Answer from the drawing. Dimensions are ordinates in mm from the lowest x, y and z of the part. Coordinates: 2 decimals unless noted, no trailing zeros. Write each loop counter-clockwise with the first axis right and the second up, starting at its lowest first coordinate (ties: lowest second). Pieces come first, ordered by that corner, then holes. Notation, with made-up numbers: (74, 28) - (131, 28) arc R17 cw to (131, 57) - close; hole circle Ø9 at (79.5, 4). An arc over 180 degrees is marked (long way). Return JSON: item names as keys, results as strings.
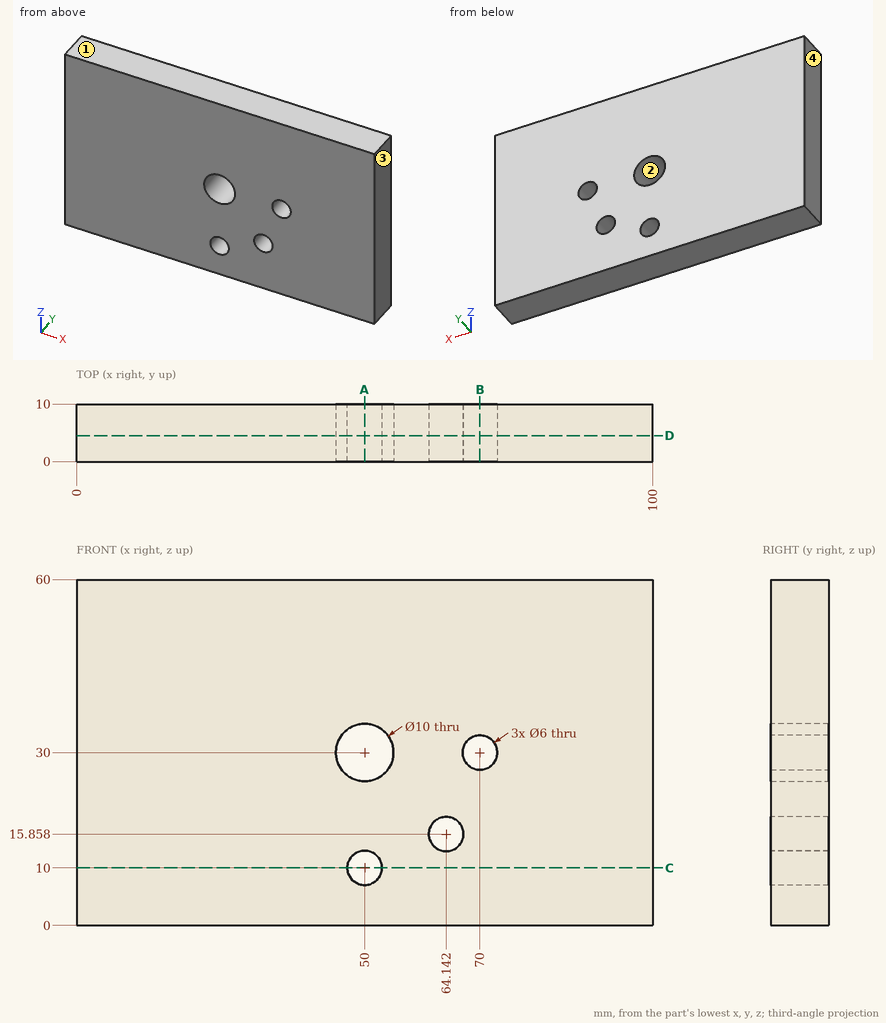
(1) Determine the mould class of the marked faces 1, 2, 3 and 4 for opening direction X: +X half, -X half, draft (parallel to the pull), parting line (faces both ways), or undercut.
Answer:
{"face 1": "draft", "face 2": "undercut", "face 3": "+X half", "face 4": "-X half"}
(2) A cutting plane is placed at D-D (y = 4.5). Determine the outline of the cut face in (x, z).
Answer:
{"outline": "(0, 0) - (100, 0) - (100, 60) - (0, 60) - close; hole circle Ø10 at (50, 30); hole circle Ø6 at (50, 10); hole circle Ø6 at (64.14, 15.86); hole circle Ø6 at (70, 30)"}
(3) A cutting plane is placed at B-B (x = 70). Determine the outline of the cut face in (y, z), and give its area (3 significant figures).
Answer:
{"outline": "(0, 0) - (10, 0) - (10, 27) - (0, 27) - close; (0, 33) - (10, 33) - (10, 60) - (0, 60) - close", "area": "540 mm²"}
(4) A cutting plane is placed at A-A (x = 50). Determine the outline of the cut face in (y, z), and give its area (3 significant figures).
Answer:
{"outline": "(0, 0) - (10, 0) - (10, 7) - (0, 7) - close; (0, 13) - (10, 13) - (10, 25) - (0, 25) - close; (0, 35) - (10, 35) - (10, 60) - (0, 60) - close", "area": "440 mm²"}
(5) Straight lines are drawn through the part: line 1 (Z direction, x = 50, y = 3.75); line 2 (X direction, y = 6.5, z = 30); line 3 (Z direction, x = 70, y = 6). For each, find the intervals that lie inside material, in ascending order. Write a range as from..to.
Answer:
{"line 1": "0..7, 13..25, 35..60", "line 2": "0..45, 55..67, 73..100", "line 3": "0..27, 33..60"}
(6) A cutting plane is placed at C-C (z = 10). Determine the outline of the cut face in (x, y), and give its area (3 significant figures).
Answer:
{"outline": "(0, 0) - (47, 0) - (47, 10) - (0, 10) - close; (53, 0) - (100, 0) - (100, 10) - (53, 10) - close", "area": "940 mm²"}
